CAD build for the part. Positions are in the model's coordinates, mm. A direction names the side the tool comes from. Round coordinates to 2 decimals unless told otherwise and drop trailing zeros. Write each loop counter-clockwise with the first axis right and the second up, starting at its lowest first coordinate (ties: lowest second). Pieces come first, ordered by that corner, then holes. Notation, with made-up numbers: (82, 50) -> (138, 50) arc R23 cw to (138, 84) -> close; hole circle Ø11 at (-32.5, -10). An arc over 180 degrees is marked (long way). Put each result on its own line as item: value. Start each with the question number.
1. Saw through at A-A on y = -25. List the corners of the cut face in (x, z), and give its area (3 significant figures).
2. 3-axis set-ups, long thin cutter, end or side, ignore diameter. For faces 1 (the flat face through (3, -20, 110)), 2 (the flat face through (0, -60, 5)), 3 (the flat face through (15, -21, 21)): which of +Z, -Z, +X, -X, +Y, -Y reach the whole face in a straight line?
3. Drill centre lines: line 1 (Z direction, x = 0, y = -13.75); line 2 (Y direction, x = 0, z = 7); line 3 (Z direction, x = -11, y = -19). Where is each one in solid material? Low to high. Write a range as from..to.
4. Saw through at D-D on z = 106.5. List the corners of the cut face in (x, y), and give its area (3 significant figures).
5. Saw through at C-C on x = -7. List the corners of the cut face in (y, z) (1 decimal), and give its area (3 significant figures).
6. Pull direction X, two halves, no side cores. Call faces 4 (the flat face through (0, -10, 66)), 5 (the cylindrical face through (22.15, -56.99, 4.93)), 6 (the flat face through (0.4, -30.4, 0)): pulls with the +X half, pulls with the -X half, needs draft (parallel to the pull), parting line crosses it, or undercut.
7. Flat gauge pins, fed straight in: P1, Ø1, axis at y = -12.5, z = 85.5, coming from the +X side; P2, Ø1.5, axis at y = -15.5, z = 77, coming from the -X side. Where does each tip first touch, or does it go through?
8. Saw through at B-B on y = -17.5. List the corners of the cut face in (x, z), and give its area (3 significant figures).
from build123d import *

# Parameters (mm, degrees)
F1_DEPTH = 25
F3_DEPTH = 10
F4_R     = 20
F5_DEPTH = 10
F6_R     = 24.99999
F8_D     = 30
F9_R     = 10
F11_D    = 10


# Not quite as in the source:
# - a fillet or chamfer is up to 0.001 mm smaller than in the source, because OpenCascade refuses the exact size
# - a pattern or mirror of a feature is missing from the dataset's text; its kind, count and spacing are read off the source's solid


with BuildPart() as f1:
    # F0 (on Right) → F1 (new body, symmetric)
    with BuildSketch(Plane.YZ):
        Polygon((-60, 0), (0, 0), (0, 120), (-10, 120), (-10, 10), (-60, 10), align=None)
    extrude(amount=F1_DEPTH, both=True)

    # F2 (on face) → F3 (join)
    with BuildSketch(Plane.YZ.offset(25)):
        Polygon((-50, 10), (-10, 10), (-10, 50), align=None)
    f3 = extrude(amount=-F3_DEPTH)

    # F3_copies: F3 across plane
    add(f3.mirror(Plane(origin=(0, 0, 0), x_dir=(0, 0, -1), z_dir=(-1, 0, 0))))

    # F4 (on face) → F5 (join)
    with BuildSketch(Plane.XZ.offset(10)):
        with Locations((0, 95)):
            Circle(F4_R)
    extrude(amount=F5_DEPTH)

    # F6 (radius 25 in the source; OpenCascade refuses exactly that, so slightly less here)
    f6_edges = [f1.edges().sort_by_distance(p)[0] for p in [
        (-25, -5, 120),
        (25, -5, 120),
    ]]
    fillet(f6_edges, radius=F6_R)

    # F8 (through all)
    with Locations(Plane.XZ.offset(20)):
        with Locations((0, 95)):
            Hole(F8_D / 2)

    # F9
    f9_edges = [f1.edges().sort_by_distance(p)[0] for p in [
        (-25, -60, 5),
        (25, -60, 5),
    ]]
    fillet(f9_edges, radius=F9_R)

    # F11 (through all)
    with Locations(Plane.XY.offset(10)):
        with Locations((0, -25), (0, -45)):
            Hole(F11_D / 2)


solid = f1.part
Return value:
1. outline: (-25, 0) -> (-5, 0) -> (-5, 10) -> (-15, 10) -> (-15, 35) -> (-25, 35) -> close; (5, 0) -> (25, 0) -> (25, 35) -> (15, 35) -> (15, 10) -> (5, 10) -> close
1. area: 900 mm^2
2. face 1: +Z, +X, -X, -Y
2. face 2: +Z, -Z, +X, -X, -Y
2. face 3: -Y
3. line 1: z = 0..10, 75..80, 110..115
3. line 2: y = -60..-50, -40..-30, -20..0
3. line 3: z = 0..10, 78.3..84.8, 105.2..111.7
4. outline: (-22.2, -10) -> (-16.36, -10) -> (-16.36, -20) -> (-9.63, -20) -> (-9.63, 0) -> (-22.2, 0) -> close; (9.63, -20) -> (16.36, -20) -> (16.36, -10) -> (22.2, -10) -> (22.2, 0) -> (9.63, 0) -> close
4. area: 386 mm^2
5. outline: (-60, 0) -> (0, 0) -> (0, 81.7) -> (-20, 81.7) -> (-20, 76.3) -> (-10, 76.3) -> (-10, 10) -> (-60, 10) -> close; (-20, 108.3) -> (0, 108.3) -> (0, 119) -> (-10, 119) -> (-10, 113.7) -> (-20, 113.7) -> close
5. area: 1,530 mm^2
6. face 4: undercut
6. face 5: pulls with the +X half
6. face 6: needs draft
7. P1: stops at x = 17.86
7. P2: stops at x = -10.12
8. outline: (-25, 0) -> (25, 0) -> (25, 42.5) -> (15, 42.5) -> (15, 10) -> (-15, 10) -> (-15, 42.5) -> (-25, 42.5) -> close; circle Ø40 at (0, 95); hole circle Ø30 at (0, 95)
8. area: 1,700 mm^2
